Geometry: final body of the model. Coordinates: model frame, mm. Face numbers are marked on the shaded views. Give positions to 0.01 mm unless a question says otherwise; leave off trailing zeros. Write each loop counter-clockwise with the first axis right and the second up, starting at its lowest first coordinate (ties: lowest second). Pieces come first, ordered by that corner, then holes. Notation, with made-up numbers: (-39.75, 86) -> (7.25, 86) arc R15 cw to (7.25, 100) -> close; hole circle Ø5 at (-26, 24). An arc over 180 degrees is marked (long way). Answer as a JSON object with one key per item and string values.
from build123d import *

# Parameters (mm, degrees)
SKETCH1_R               = 14.5
SKETCH1_R_2             = 6
BOSS_EXTRUDE1_DEPTH     = 1
BOSS_EXTRUDE2_START     = -3
BOSS_EXTRUDE2_DEPTH     = 3
CUT_EXTRUDE1_DEPTH      = 24.526580712
CUT_EXTRUDE1_DEPTH_BACK = 24.526580712
SKETCH3_W               = 29
SKETCH3_H               = 5.5


with BuildPart() as part:
    # Sketch1 → Boss-Extrude1 (new body)
    # profile 1 of 3: a face of its own
    with BuildSketch(Plane(origin=(0, 0, 0), x_dir=(1, 0, 0), z_dir=(0, 1, 0))):
        Circle(SKETCH1_R)
        with Locations(Location((0, 0, 0), (0, 0, 270))):
            Circle(SKETCH1_R_2, mode=Mode.SUBTRACT)
    # profile 2 of 3: a face of its own
    with BuildSketch(Plane(origin=(0, 0, 0), x_dir=(1, 0, 0), z_dir=(0, 1, 0))):
        with BuildLine():
            ThreePointArc((0, -14.5), (-10.253048327, -10.253048327), (-14.5, 0))
            Line((-14.5, 0), (-14.5, -14.5))
            Line((-14.5, -14.5), (0, -14.5))
        make_face()
    # profile 3 of 3: a face of its own
    with BuildSketch(Plane(origin=(0, 0, 0), x_dir=(1, 0, 0), z_dir=(0, 1, 0))):
        with BuildLine():
            Line((14.5, -14.5), (14.5, 0))
            ThreePointArc((14.5, 0), (10.253048327, -10.253048327), (0, -14.5))
            Line((0, -14.5), (14.5, -14.5))
        make_face()
    extrude(amount=BOSS_EXTRUDE1_DEPTH)

    # Sketch2 → Boss-Extrude2 (add)
    with BuildSketch(Plane(origin=(0, 1, 0), x_dir=(1, 0, 0), z_dir=(0, 1, 0)).offset(BOSS_EXTRUDE2_START)):
        with BuildLine():
            ThreePointArc((7.874007874, -14.5), (4.062019223, -15.992185587), (4.2e-08, -16.5))
            Line((4.2e-08, -16.5), (16.5, -16.5))
            Line((16.5, -16.5), (16.5, 0))
            ThreePointArc((16.5, 0), (15.992185592, -4.062019202), (14.5, -7.874007874))
            Line((14.5, -7.874007874), (14.5, -14.5))
            Line((14.5, -14.5), (7.874007874, -14.5))
        make_face()
        with BuildLine():
            ThreePointArc((-7.874007874, -14.5), (-4.062019182, -15.992185597), (4.2e-08, -16.5))
            ThreePointArc((4.2e-08, -16.5), (4.062019223, -15.992185587), (7.874007874, -14.5))
            Line((7.874007874, -14.5), (-7.874007874, -14.5))
        make_face()
        with BuildLine():
            ThreePointArc((-14.5, -7.874007874), (-15.992185592, -4.062019202), (-16.5, 0))
            Line((-16.5, 0), (-16.5, -16.5))
            Line((-16.5, -16.5), (4.2e-08, -16.5))
            ThreePointArc((4.2e-08, -16.5), (-4.062019182, -15.992185597), (-7.874007874, -14.5))
            Line((-7.874007874, -14.5), (-14.5, -14.5))
            Line((-14.5, -14.5), (-14.5, -7.874007874))
        make_face()
        with BuildLine():
            Line((-14.5, 0), (-16.5, 0))
            ThreePointArc((-16.5, 0), (-15.992185592, -4.062019202), (-14.5, -7.874007874))
            Line((-14.5, -7.874007874), (-14.5, 0))
        make_face()
        with BuildLine():
            Line((16.5, 0), (14.5, 0))
            Line((14.5, 0), (14.5, -7.874007874))
            ThreePointArc((14.5, -7.874007874), (15.992185592, -4.062019202), (16.5, 0))
        make_face()
        with BuildLine():
            ThreePointArc((3.4e-08, 16.5), (-11.667261877, 11.667261902), (-16.5, 0))
            Line((-16.5, 0), (-14.5, 0))
            ThreePointArc((-14.5, 0), (0, 14.5), (14.5, 0))
            Line((14.5, 0), (16.5, 0))
            ThreePointArc((16.5, 0), (11.667261902, 11.667261877), (3.4e-08, 16.5))
        make_face()
    extrude(amount=BOSS_EXTRUDE2_DEPTH)

    # Sketch3 → Cut-Extrude1 (cut, two sides: drawn at the far end of the back side and taken through both)
    with BuildSketch(Plane.XZ.offset(2).offset(-CUT_EXTRUDE1_DEPTH_BACK)):
        Polygon((16.5, 16.5), (-16.5, 16.5), (-16.5, 9), (-14.5, 9), (-14.5, 14.5), (14.5, 14.5), (14.5, 9), (16.5, 9), align=None)
        with Locations((0, 11.75)):
            Rectangle(SKETCH3_W, SKETCH3_H)
    extrude(amount=CUT_EXTRUDE1_DEPTH + CUT_EXTRUDE1_DEPTH_BACK, mode=Mode.SUBTRACT)


solid = part.part
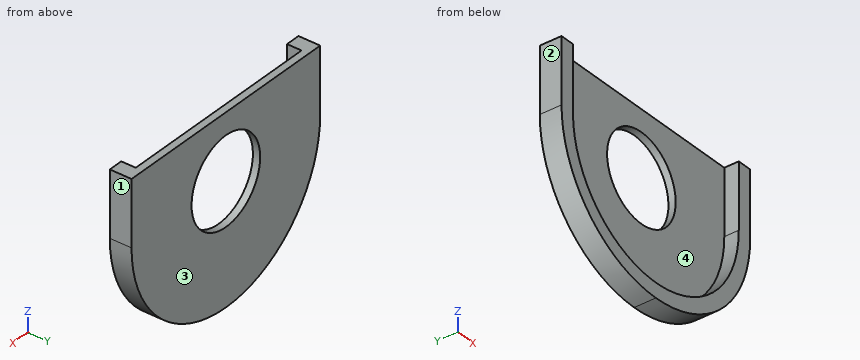
Q1. Cut plane B-B (x = 5). Return the cut outline in (y, z).
Values:
{"outline": "(-2, -15.72) -> (1, -15.72) -> (1, -3.32) -> (0, -3.32) -> (0, -13.61) -> (-2, -13.61) -> close; (0, 3.32) -> (1, 3.32) -> (1, 9) -> (0, 9) -> close"}
Q2. Material intervals for L1, parallel to X at y = -0.15, z = 6; L2, parallel to X at y = 0.4, z = 0; L3, parallel to Y at x = 12, z = 6, sorted ascending. Write a range as from..to.
Values:
{"L1": "-16.5..-14.5, 14.5..16.5", "L2": "-16.5..-6, 6..16.5", "L3": "0..1"}
Q3. First-contact query: P1, Ø5, axis at x = -6, z = -2, coming from the -Y side. Flat tip, straight axial feed; report the tip coordinate or a pass-through.
Values:
{"P1": "y = 0"}
Q4. Cut plane D-D (x = -7). Return the cut outline in (y, z).
Values:
{"outline": "(-2, -14.94) -> (1, -14.94) -> (1, 9) -> (0, 9) -> (0, -12.7) -> (-2, -12.7) -> close"}
Q5. Cut plane C-C (z = -5.25). Return the cut outline in (x, y), and give its area (3 significant figures).
Values:
{"outline": "(-15.64, -2) -> (-13.52, -2) -> (-13.52, 0) -> (-2.9, 0) -> (-2.9, 1) -> (-15.64, 1) -> close; (2.9, 0) -> (13.52, 0) -> (13.52, -2) -> (15.64, -2) -> (15.64, 1) -> (2.9, 1) -> close", "area": "34.0 mm²"}
Q6. Mould query, pull axis X, two halves, no side actions, for the marked faces 1, 2, 3 and 4. Classes: pulls with the +X half, pulls with the -X half, needs draft (parallel to the pull), parting line crosses it, or undercut.
Values:
{"face 1": "pulls with the +X half", "face 2": "pulls with the -X half", "face 3": "needs draft", "face 4": "undercut"}
Q7. Cut plane A-A (y = -0.5). Return the cut outline in (x, z), and give its area (3 significant figures).
Values:
{"outline": "(-16.5, 0) arc R16.5 ccw to (16.5, 0) -> (16.5, 9) -> (14.5, 9) -> (14.5, 0) arc R14.5 cw to (-14.5, 0) -> (-14.5, 9) -> (-16.5, 9) -> close", "area": "133 mm²"}
